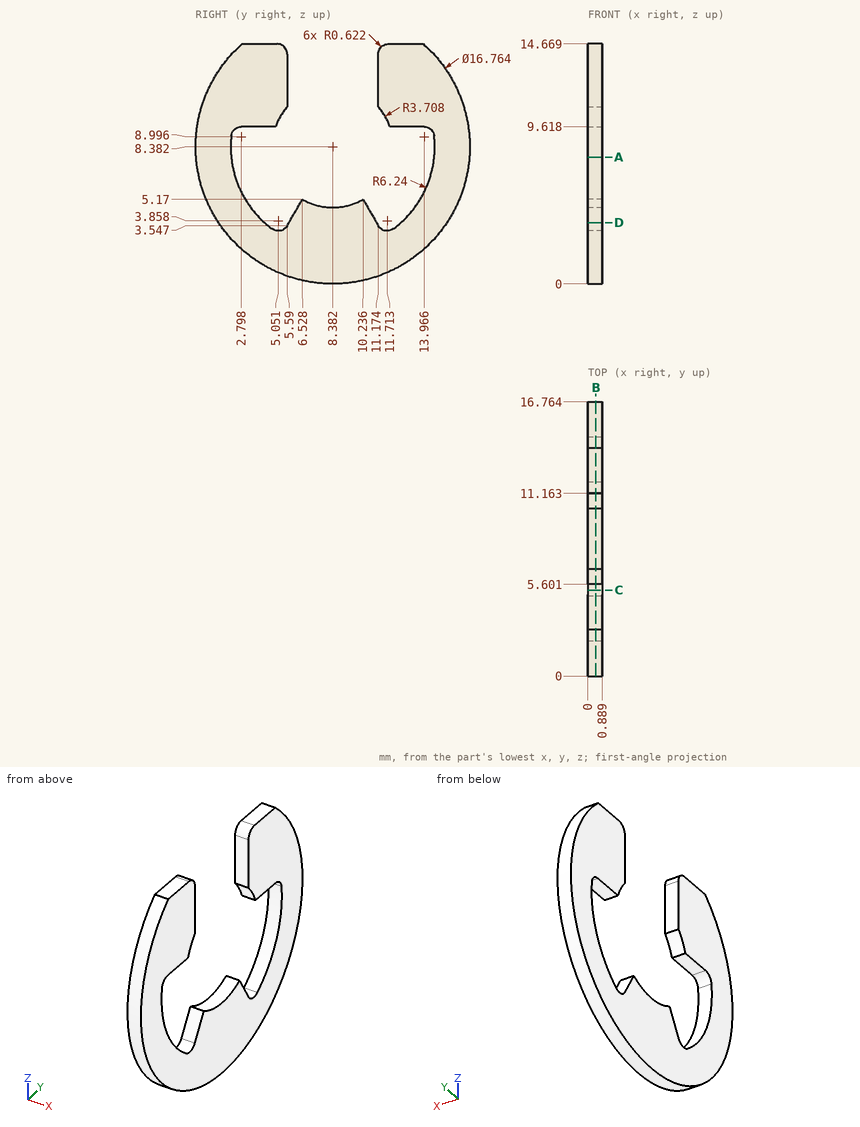
Input: dimensioned drawing with shaded views. Units: mm. Origin: part minimum x, y, z. Give positions to 0.01 mm unless a question says otherwise; leave off trailing zeros. Loops run counter-clockwise (first coordinate to the right, second up) from the corner with the lowest first, then second, coordinate; pieces in that order, holes last. Notation, with made-up numbers: (38.5, 2) -> (95.5, 2) arc R23 cw to (95.5, 20) -> close; hole circle Ø6 at (23, -35). An arc over 180 degrees is marked (long way). Use a Markdown table: item, result.
Q1. Section query D-D, the plane z = 3.75. Return the cut outline in (x, y).
Entries:
| item | result |
|---|---|
| outline | (0, 1.4) -> (0.89, 1.4) -> (0.89, 4.2) -> (0, 4.2) -> close; (0, 5.71) -> (0.89, 5.71) -> (0.89, 11.06) -> (0, 11.06) -> close; (0, 12.56) -> (0.89, 12.56) -> (0.89, 15.37) -> (0, 15.37) -> close |
Q2. Section query B-B, the plane x = 0.5. Return the cut outline in (y, z) (1 decimal).
Entries:
| item | result |
|---|---|
| outline | (2.2, 9.1) arc R0.6 cw to (2.8, 9.6) -> (4.9, 9.6) arc R3.7 cw to (5.6, 10.8) -> (5.6, 14) arc R0.6 ccw to (5, 14.7) -> (2.8, 14.7) arc R8.4 ccw (long way) to (13.9, 14.7) -> (11.8, 14.7) arc R0.6 ccw to (11.2, 14) -> (11.2, 10.8) arc R3.7 cw to (11.9, 9.6) -> (14, 9.6) arc R0.6 cw to (14.6, 9.1) arc R6.2 cw to (12.1, 3.4) arc R0.6 cw to (11.2, 3.5) -> (10.2, 5.2) arc R3.7 cw to (6.5, 5.2) -> (5.6, 3.5) arc R0.6 cw to (4.7, 3.4) arc R6.2 cw to start |
Q3. Ray query, probe 1 along Y at (x, z) = (0.25, 3.75) (1 decimal); probe 2 along Y at (x, z) = (0.3, 14.25) (1 decimal); probe 3 along Y at (x, z) = (0.4, 8.5). Return the intervals inside material, ascending. Write a range as from..to.
Entries:
| item | result |
|---|---|
| probe 1 | y = 1.4..4.2, 5.7..11.1, 12.6..15.4 |
| probe 2 | y = 2.4..5.6, 11.2..14.4 |
| probe 3 | y = 0..2.14, 14.62..16.76 |
Q4. Section query C-C, the plane y = 5.25. Return the cut outline in (x, z).
Entries:
| item | result |
|---|---|
| outline | (0, 0.61) -> (0.89, 0.61) -> (0.89, 3.27) -> (0, 3.27) -> close; (0, 10.37) -> (0.89, 10.37) -> (0.89, 14.61) -> (0, 14.61) -> close |
Q5. First-contact query: P1, Ø4, axis at y = 10.5, z = 8.5, coming from the +X side. Flat tip, straight axial feed; report the tip coordinate or a pass-through.
Entries:
| item | result |
|---|---|
| P1 | stops at x = 0.89 |
Q6. Section query A-A, the plane z = 7.75. Return the cut outline in (x, y).
Entries:
| item | result |
|---|---|
| outline | (0, 0.02) -> (0.89, 0.02) -> (0.89, 2.17) -> (0, 2.17) -> close; (0, 14.59) -> (0.89, 14.59) -> (0.89, 16.74) -> (0, 16.74) -> close |
